Here's how the part is built. I have some questions about the finished solid (model axes, mm). A direction names the side the tool comes from. Round coordinates to 2 decimals unless told otherwise and drop trailing zeros. Write each loop counter-clockwise with the first axis right and the second up, starting at its lowest first coordinate (ties: lowest second). Pieces come first, ordered by that corner, then holes. Notation, with made-up numbers: (36.25, 19) -> (60.25, 19) arc R12 ccw to (60.25, 26) -> close; hole circle Ø10 at (51, 85.25). An arc over 180 degrees is marked (long way). Put each result on its own line as item: value. Start each with the question number.
1. For pin 1 (5 mm diameter, centred on x = 27.5, z = -17, fed in from -Y); pin 2 (2.5 mm diameter, centred on x = 30, z = -4, fed in from +Y); pin 3 (1 mm diameter, centred on y = 13, z = -10, fed in from +X); pin 4 (0.6 mm diameter, centred on x = -35.5, z = -4, fed in from +Y), each with a flat end and sliding along its axis, tell me the tip position at first contact or that it passes through.
2. Suppose I cut it at D-D (y = 22.5). Please give me the cut outline in (x, z), then the cut area to 3 significant figures.
3. Suppose I cut it at B-B (z = -13). Please give me the cut outline in (x, y), then the cut area to 3 significant figures.
4. Suppose I cut it at C-C (x = -22.5). Please give me the cut outline in (y, z), then the cut area to 3 significant figures.
5. I need wall thicknesses on probe 1 along X at (y, z) = (3.9, 2); probe 2 along Z at (x, y) = (-42.5, 20.5); probe 3 along Z at (x, y) = (-9.5, 13.75). Which ranges of each line are inside material? Lowest first, please. Write a range as from..to.
6. Which directions (+Z, -Z, +X, -X, +Y, -Y) give clear straight access to the entire face, cutting with the end or side of a thin tool? Please do faces 1 (the face through (22.175, 1.521, 27.139)), 2 (the face through (47.8, 3, -2.4)), 3 (the face through (-1, 14, -36)), 4 (the face through (43, 9, -11.164)).
7. We'd pull the mould along X, two halves only. Please class faces 5 (the face through (32, 4.78, -4.32)), 6 (the face through (31.97, 4.78, 2.4)), 7 (the face through (43, 15, -18)), 8 (the face through (45, 12, 1)): +X half, -X half, draft (parallel to the pull), parting line (faces both ways), or undercut.
8. Suppose I cut it at A-A (y = 5). Count the separate pieces of the cut face and the enclosed holes in it, then the cut area to 3 significant figures.
```python
from build123d import *

# Parameters (mm, degrees)
SKETCH1_R           = 2.495486553
BOSS_EXTRUDE1_DEPTH = 3
SKETCH2_R           = 2.5
BOSS_EXTRUDE2_DEPTH = 4
SKETCH3_R           = 1.5
CUT_EXTRUDE1_DEPTH  = 3
SKETCH4_R           = 1.05
CUT_EXTRUDE2_DEPTH  = 4.5
SKETCH6_W           = 90
SKETCH6_H           = 80
SKETCH6_W_2         = 82
SKETCH6_H_2         = 72
BOSS_EXTRUDE3_DEPTH = 22
SKETCH7_W           = 13.75
SKETCH7_H           = 12
CUT_EXTRUDE3_DEPTH  = 20
SKETCH8_R           = 1.5
CUT_EXTRUDE4_DEPTH  = 10
SKETCH10_W          = 6.5
SKETCH10_H          = 5.005531991
CUT_EXTRUDE5_DEPTH  = 10


with BuildPart() as part:
    # Sketch1 → Boss-Extrude1 (new body)
    with BuildSketch(Plane(origin=(0, 0, 0), x_dir=(1, 0, 0), z_dir=(0, 1, 0))):
        with BuildLine():
            Line((-45, 40), (-10, 40))
            Line((-10, 40), (10, 40))
            Line((10, 40), (45, 40))
            Line((45, 40), (45, 10))
            ThreePointArc((45, 10), (55, 0), (45, -10))
            Line((45, -10), (45, -40))
            Line((45, -40), (10, -40))
            Line((10, -40), (-10, -40))
            Line((-10, -40), (-45, -40))
            Line((-45, -40), (-45, -10))
            ThreePointArc((-45, -10), (-55, 0), (-45, 10))
            Line((-45, 10), (-45, 40))
        make_face()
        with Locations((-49, 0)):
            Circle(SKETCH1_R, mode=Mode.SUBTRACT)
        with Locations((49, 0)):
            Circle(SKETCH1_R, mode=Mode.SUBTRACT)
    extrude(amount=BOSS_EXTRUDE1_DEPTH)

    # Sketch2 → Boss-Extrude2 (add)
    with BuildSketch(Plane(origin=(0, 3, 0), x_dir=(1, 0, 0), z_dir=(0, 1, 0))):
        with Locations((-35, 30)):
            Circle(SKETCH2_R)
        with Locations((31, 30)):
            Circle(SKETCH2_R)
        with Locations((31, 4)):
            Circle(SKETCH2_R)
        with Locations((-35, 4)):
            Circle(SKETCH2_R)
        with Locations((-35, -2)):
            Circle(SKETCH2_R)
        with Locations((31, -2)):
            Circle(SKETCH2_R)
        with Locations((-35, -15)):
            Circle(SKETCH2_R)
        with Locations((31, -15)):
            Circle(SKETCH2_R)
    extrude(amount=BOSS_EXTRUDE2_DEPTH)

    # Sketch3 → Cut-Extrude1 (cut)
    with BuildSketch(Plane(origin=(0, 3, 0), x_dir=(1, 0, 0), z_dir=(0, 1, 0))):
        with Locations((-22.5, -25.674226477)):
            Circle(SKETCH3_R)
        with Locations((22.5, -25.674226477)):
            Circle(SKETCH3_R)
    extrude(amount=-CUT_EXTRUDE1_DEPTH, mode=Mode.SUBTRACT)

    # Sketch4 → Cut-Extrude2 (cut)
    with BuildSketch(Plane(origin=(0, 7, 0), x_dir=(1, 0, 0), z_dir=(0, 1, 0))):
        with Locations((-35, 30)):
            Circle(SKETCH4_R)
        with Locations((31, 30)):
            Circle(SKETCH4_R)
        with Locations((31, 4)):
            Circle(SKETCH4_R)
        with Locations((31, -2)):
            Circle(SKETCH4_R)
        with Locations((-35, 4)):
            Circle(SKETCH4_R)
        with Locations((-35, -2)):
            Circle(SKETCH4_R)
        with Locations((-35, -15)):
            Circle(SKETCH4_R)
        with Locations((31, -15)):
            Circle(SKETCH4_R)
    extrude(amount=-CUT_EXTRUDE2_DEPTH, mode=Mode.SUBTRACT)

    # Sketch6 → Boss-Extrude3 (add)
    with BuildSketch(Plane(origin=(0, 3, 0), x_dir=(1, 0, 0), z_dir=(0, 1, 0))):
        Rectangle(SKETCH6_W, SKETCH6_H)
        Rectangle(SKETCH6_W_2, SKETCH6_H_2, mode=Mode.SUBTRACT)
    extrude(amount=BOSS_EXTRUDE3_DEPTH)

    # Sketch7 → Cut-Extrude3 (cut)
    with BuildSketch(Plane.ZY.offset(-41)):
        with Locations((-18.038625802, 9)):
            Rectangle(SKETCH7_W, SKETCH7_H)
    extrude(amount=-CUT_EXTRUDE3_DEPTH, mode=Mode.SUBTRACT)

    # Sketch8 → Cut-Extrude4 (cut)
    with BuildSketch(Plane(origin=(0, 25, 0), x_dir=(1, 0, 0), z_dir=(0, 1, 0))):
        with Locations((-42.5, 37.5)):
            Circle(SKETCH8_R)
        with Locations((42.5, 37.5)):
            Circle(SKETCH8_R)
        with Locations((-42.5, -38)):
            Circle(SKETCH8_R)
        with Locations((42.5, -37.5)):
            Circle(SKETCH8_R)
    extrude(amount=-CUT_EXTRUDE4_DEPTH, mode=Mode.SUBTRACT)

    # Sketch10 → Cut-Extrude5 (cut)
    with BuildSketch(Plane(origin=(-41, 0, 0), x_dir=(0, 0, -1), z_dir=(1, 0, 0))):
        with Locations((-8.55, 5.502765995)):
            Rectangle(SKETCH10_W, SKETCH10_H)
    extrude(amount=-CUT_EXTRUDE5_DEPTH, mode=Mode.SUBTRACT)


solid = part.part
```
Verdict:
1. pin 1: stops at y = 0
1. pin 2: stops at y = 7
1. pin 3: stops at x = 45
1. pin 4: stops at y = 2.5
2. outline: (-45, -40) -> (45, -40) -> (45, 40) -> (-45, 40) -> close; hole circle Ø3 at (-42.5, -37.5); hole circle Ø3 at (-42.5, 38); hole (-41, -36) -> (41, -36) -> (41, 36) -> (-41, 36) -> close; hole circle Ø3 at (42.5, -37.5); hole circle Ø3 at (42.5, 37.5)
2. area: 1,270 mm^2
3. outline: (-45, 0) -> (45, 0) -> (45, 3) -> (-41, 3) -> (-41, 25) -> (-45, 25) -> close; (41, 15) -> (45, 15) -> (45, 25) -> (41, 25) -> close
3. area: 398 mm^2
4. outline: (0, -40) -> (25, -40) -> (25, -36) -> (3, -36) -> (3, 24.17) -> (0, 24.17) -> close; (0, 27.17) -> (3, 27.17) -> (3, 36) -> (25, 36) -> (25, 40) -> (0, 40) -> close
4. area: 407 mm^2
5. probe 1: x = -45..-41, -37.5..-36.05, -33.95..-32.5, 28.5..29.95, 32.05..33.5, 41..45
5. probe 2: z = -40..-39, -36..36.5, 39.5..40
5. probe 3: z = -40..-36, 36..40
6. face 1: +Y, -Y
6. face 2: +Z, -Z, +X, +Y
6. face 3: +Y
6. face 4: +X
7. face 5: undercut
7. face 6: undercut
7. face 7: draft
7. face 8: +X half
8. separate pieces: 10
8. enclosed holes: 8
8. area: 1,340 mm^2
